Verification items for this drawing (mm, ordinates from the low corner). Coordinates: 2 decimals unless noted, no trailing zeros. Loops run counter-clockwise (first coordinate to the right, second up) from the corner with the lowest first, then second, coordinate; pieces in that order, holes last. Notation, with made-up numbers: (89.5, 2) - (143.5, 2) arc R33 cw to (143.5, 33) - close; hole circle Ø3 at (17, 26.25). An arc over 180 degrees is marked (long way). One line per item, written item: value. Start each with the question number.
(1) Section check C-C (z = 0.55). Record the boundary of the cut face in (x, y), plus the area to 3 significant figures.
(2) Section check B-B (x = 5). Record the boundary of the cut face in (y, z), plus the area to 3 significant figures.
(3) Section check D-D (y = 9.25). Record the boundary of the cut face in (x, z).
(4) Draft check along X on the marked faces 1, 2 and 3. Enter one of: +X half, -X half, draft (parallel to the pull), parting line (faces both ways), or undercut.
(5) Thickness scan on probe 1 along Y at (x, z) = (5, 0.5); probe 2 along X at (y, z) = (2, 1.15); probe 3 along X at (y, z) = (15.25, 0.55). Record the ranges inside material, lowest first. Write a range as [from, to].
(6) Section check A-A (y = 2). Record the boundary of the cut face in (x, z).
(7) Gauge pin test, flat end, axial feed: P1, Ø1.8, axis at x = 5, y = 16.5, coming from the +Z side. Record the tip position at first contact, or that the pin passes through.
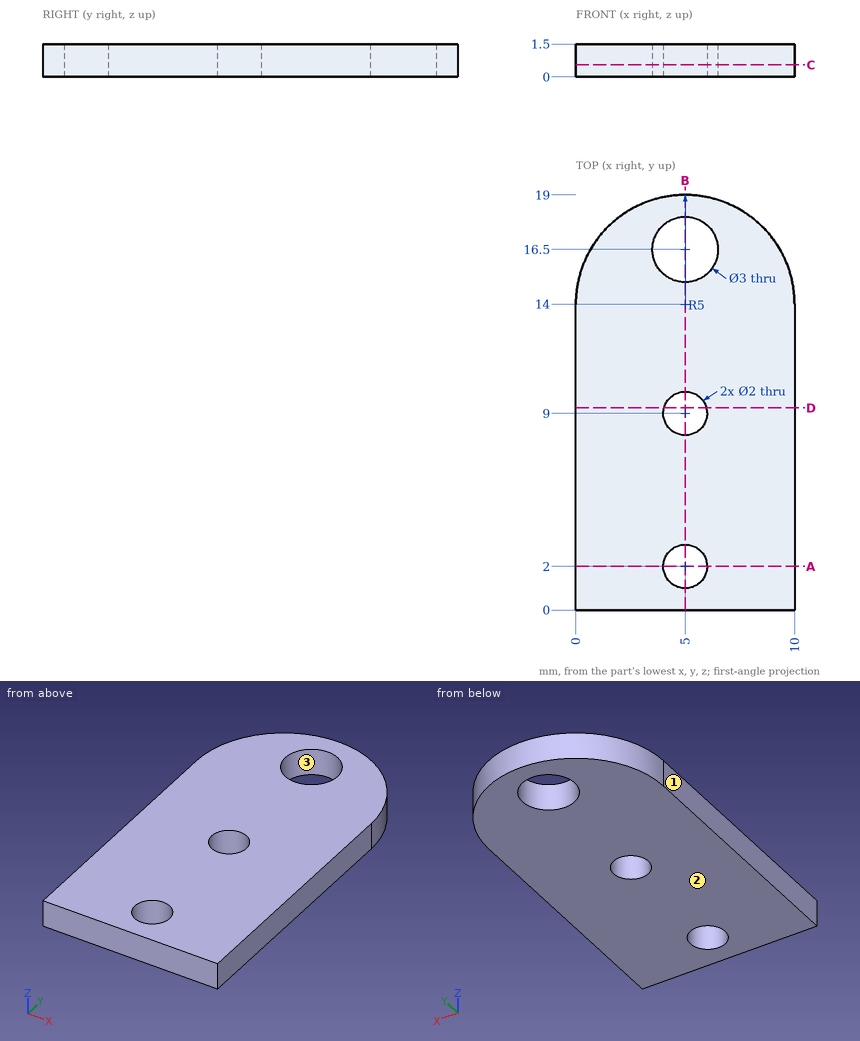
Responses:
1. outline: (0, 0) - (10, 0) - (10, 14) arc R5 ccw to (0, 14) - close; hole circle Ø3 at (5, 16.5); hole circle Ø2 at (5, 2); hole circle Ø2 at (5, 9)
1. area: 166 mm²
2. outline: (0, 0) - (1, 0) - (1, 1.5) - (0, 1.5) - close; (3, 0) - (8, 0) - (8, 1.5) - (3, 1.5) - close; (10, 0) - (15, 0) - (15, 1.5) - (10, 1.5) - close; (18, 0) - (19, 0) - (19, 1.5) - (18, 1.5) - close
2. area: 18.0 mm²
3. outline: (0, 0) - (4.03, 0) - (4.03, 1.5) - (0, 1.5) - close; (5.97, 0) - (10, 0) - (10, 1.5) - (5.97, 1.5) - close
4. face 1: -X half
4. face 2: draft
4. face 3: undercut
5. probe 1: y = [0, 1], [3, 8], [10, 15], [18, 19]
5. probe 2: x = [0, 4], [6, 10]
5. probe 3: x = [0.16, 4.17], [5.83, 9.84]
6. outline: (0, 0) - (4, 0) - (4, 1.5) - (0, 1.5) - close; (6, 0) - (10, 0) - (10, 1.5) - (6, 1.5) - close
7. P1: passes through
